Could you check a few things on this drawing? It's one solid part, dimensions in mm from its lowest x, y, z. A direction names the side the tool comes from. Give positions to 0.01 mm unless a question says otherwise; leave off trailing zeros. Loops run counter-clockwise (first coordinate to the right, second up) from the corner with the lowest first, then second, coordinate; pieces in that order, holes last. Notation, with made-up numbers: (64.25, -36.5) - (68.25, -36.5) arc R5 cw to (68.25, -30.5) - close; hole circle Ø1 at (43.25, 40.5). An arc over 180 degrees is marked (long way). One line per item, written item: value. Start each with the question number.
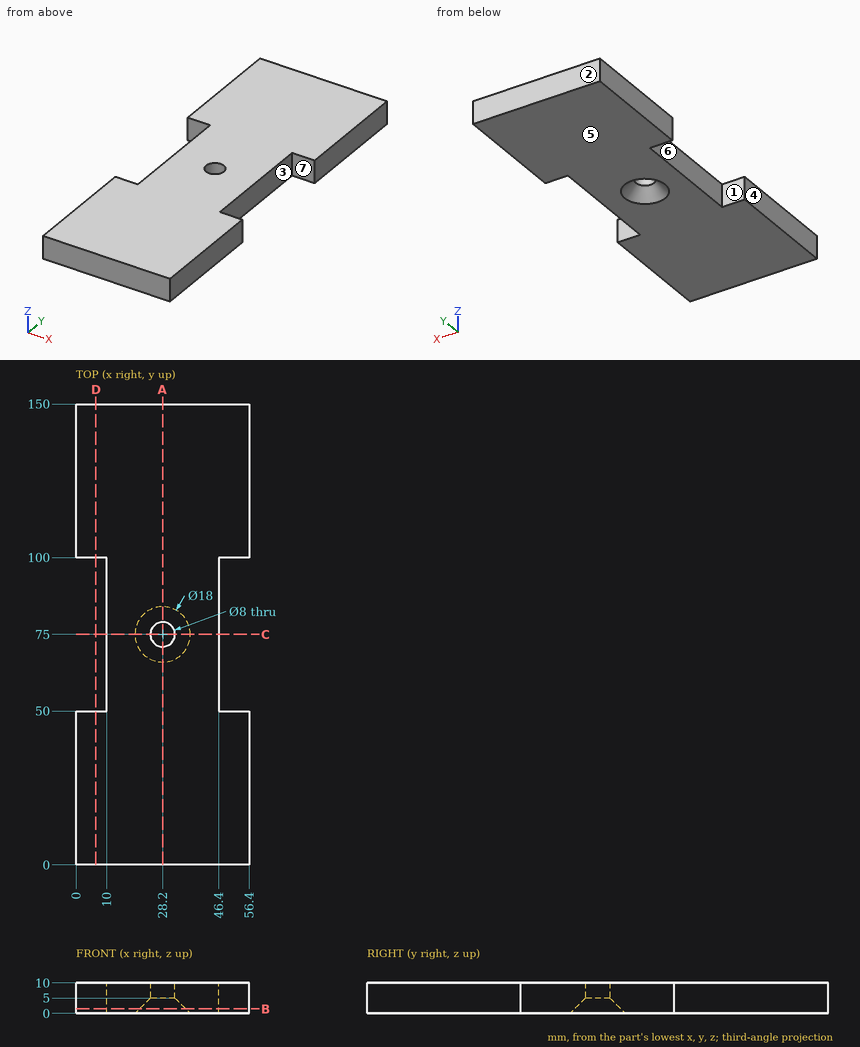
(1) Please list where these lines run through material, in increasing order: probe 1 along Y at (x, z) = (28.2, 6.4); probe 2 along Y at (x, z) = (53.5, 7); probe 3 along X at (y, z) = (57, 3.25). Write a range as from..to.
(2) If we mould it in two halves opening along Y, with no side actions, what happens to the marked faces 1, 2, 3 and 4? For each: pulls with the +Y half, pulls with the -Y half, needs draft (parallel to the pull), parting line crosses it, or undercut.
(3) If we section it at C-C on y = 75: List the corners of the cut face in (x, z) for me.
(4) Will these pins go through, and if not, where does the flat tip stop? pin 1 (3 mm diameter, centred on y = 82.5, z = 7.5, fed in from -X); pin 2 (10.5 mm diameter, centred on x = 28.2, y = 75, fed in from -Z); pin 3 (5 mm diameter, centred on y = 85, z = 4, fed in from +X).
(5) If we section it at B-B on z = 1.5: List the corners of the cut face in (x, y) for me.
(6) If we section it at A-A on x = 28.2: List the corners of the cut face in (y, z) for me.
(7) For the marked faces 5, 6 and 7, which set-ups out of +Z, -Z, +X, -X, +Y, -Y let a thin tool reach every point of the face, with its end or its side?
(8) If we section it at D-D on x = 6.5: List the corners of the cut face in (y, z) for me.
Found:
1. probe 1: 0..71, 79..150
1. probe 2: 0..50, 100..150
1. probe 3: 10..46.4
2. face 1: undercut
2. face 2: pulls with the +Y half
2. face 3: undercut
2. face 4: needs draft
3. outline: (10, 0) - (19.2, 0) - (24.2, 5) - (24.2, 10) - (10, 10) - close; (32.2, 5) - (37.2, 0) - (46.4, 0) - (46.4, 10) - (32.2, 10) - close
4. pin 1: x = 10
4. pin 2: z = 3.75
4. pin 3: x = 46.4
5. outline: (0, 0) - (56.4, 0) - (56.4, 50) - (46.4, 50) - (46.4, 100) - (56.4, 100) - (56.4, 150) - (0, 150) - (0, 100) - (10, 100) - (10, 50) - (0, 50) - close; hole circle Ø15 at (28.2, 75)
6. outline: (0, 0) - (66, 0) - (71, 5) - (71, 10) - (0, 10) - close; (79, 5) - (84, 0) - (150, 0) - (150, 10) - (79, 10) - close
7. face 5: -Z, +X, -X, +Y, -Y
7. face 6: +Z, -Z, -X
7. face 7: +Z, -Z, +X
8. outline: (0, 0) - (50, 0) - (50, 10) - (0, 10) - close; (100, 0) - (150, 0) - (150, 10) - (100, 10) - close
